Drawing for the job (mm, zero at the part's lowest x, y, z). Round coordinates to 2 decimals unless told otherwise and drop trailing zeros. Write each loop counter-clockwise with the first axis right and the second up, starting at its lowest first coordinate (ties: lowest second). Pieces come first, ordered by that corner, then holes. Notation, with made-up numbers: M 23,41 L 61,41 A18 cw 61,50 Z; hole C 2,-22 d7. An arc over 180 degrees is marked long. Use a Markdown table: item, result.
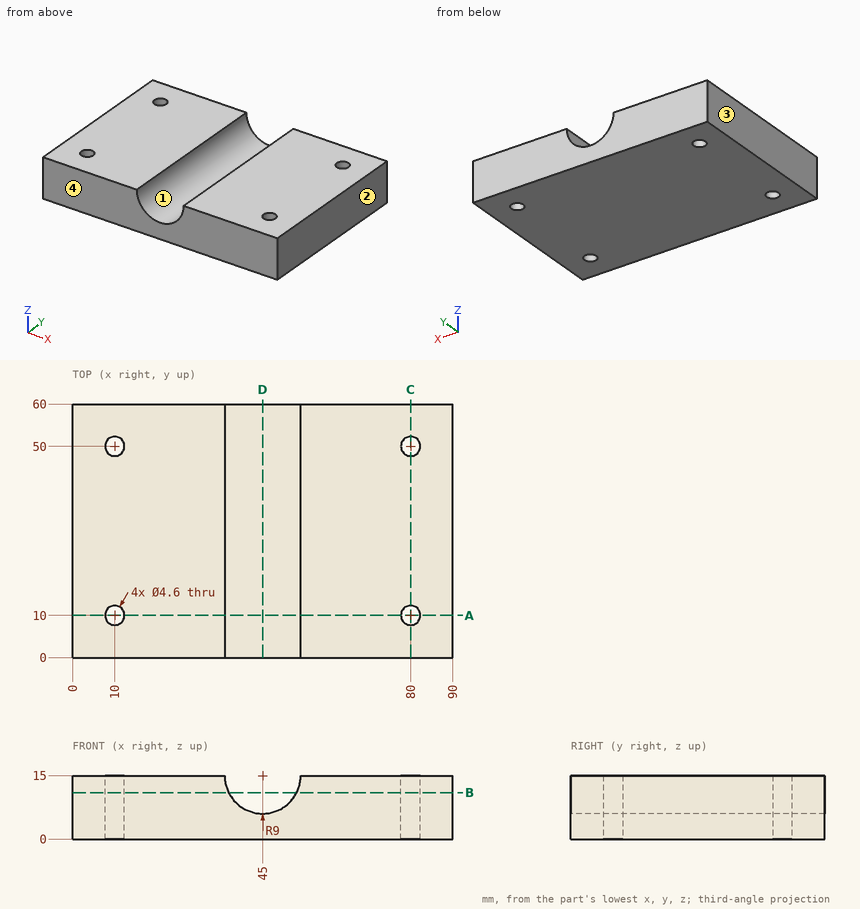
Q1. Cut at A-A on y = 10. Give the cut face in (x, z).
Response values:
| item | result |
|---|---|
| outline | M 0,0 L 7.7,0 L 7.7,15 L 0,15 Z; M 12.3,0 L 77.7,0 L 77.7,15 L 54,15 A9 cw 36,15 L 12.3,15 Z; M 82.3,0 L 90,0 L 90,15 L 82.3,15 Z |
Q2. Cut at D-D on x = 45. Give the cut face in (y, z), and give its area (3 significant figures).
Response values:
| item | result |
|---|---|
| outline | M 0,0 L 60,0 L 60,6 L 0,6 Z |
| area | 360 mm2 |
Q3. Two-plate mould, pull along X, no slides. Class the marked faces 1, 2, 3 and 4: +X half, -X half, draft (parallel to the pull), parting line (faces both ways), or undercut.
Response values:
| item | result |
|---|---|
| face 1 | undercut |
| face 2 | +X half |
| face 3 | -X half |
| face 4 | draft |
Q4. Drill centre lines: L1, parallel to Y at x = 80, z = 10; L2, parallel to X at y = 8.5, z = 10; L3, parallel to Y at x = 10.5, z = 7.75 (3 decimals). Where is each one in solid material? Low to high.
Response values:
| item | result |
|---|---|
| L1 | y = 0 to 7.7, 12.3 to 47.7, 52.3 to 60 |
| L2 | x = 0 to 8.26, 11.74 to 37.52, 52.48 to 78.26, 81.74 to 90 |
| L3 | y = 0 to 7.755, 12.245 to 47.755, 52.245 to 60 |
Q5. Cut at B-B on z = 11. Give the cut face in (x, y), and give its area (3 significant figures).
Response values:
| item | result |
|---|---|
| outline | M 0,0 L 36.94,0 L 36.94,60 L 0,60 Z; M 53.06,0 L 90,0 L 90,60 L 53.06,60 Z; hole C 10,10 d4.6; hole C 10,50 d4.6; hole C 80,10 d4.6; hole C 80,50 d4.6 |
| area | 4,370 mm2 |
Q6. Cut at C-C on x = 80. Give the cut face in (y, z), and give its area (3 significant figures).
Response values:
| item | result |
|---|---|
| outline | M 0,0 L 7.7,0 L 7.7,15 L 0,15 Z; M 12.3,0 L 47.7,0 L 47.7,15 L 12.3,15 Z; M 52.3,0 L 60,0 L 60,15 L 52.3,15 Z |
| area | 762 mm2 |
